The model under review builds one solid part; all positions refer to its coordinate system, in mm. A direction names the side the tool comes from. Coordinates: 2 decimals unless noted, no trailing zeros. Loops run counter-clockwise (first coordinate to the right, second up) from the corner with the lowest first, then second, coordinate; pieces in that order, holes last. Notation, with made-up numbers: M -29,49.5 L -10,49.5 A22 ccw -10,72.5 Z; hole C 70,-9 d8. An arc over 180 degrees is marked long. Use CSV: the item, a comma, the result in double quotes. Start each with the question number.
Autodesk Inventor part; units mm, degrees
ref_plane "YZ Plane" through (0, 0, 0) normal (1, 0, 0) x (0, 1, 0)
ref_plane "XZ Plane" through (0, 0, 0) normal (0, 1, 0) x (-1, 0, 0)
ref_plane "XY Plane" through (0, 0, 0) normal (0, 0, 1) x (1, 0, 0)
sketch "スケッチ1" plane through (0, 0, 0) normal (0, 0, 1) x (1, 0, 0)
  line L0 (-28, -52.5) -> (28, -52.5) construction
  line L1 (28, -52.5) -> (28, 52.5) construction
  line L2 (28, 52.5) -> (-28, 52.5) construction
  line L3 (-28, 52.5) -> (-28, -52.5) construction
  line L4 (-28, -52.5) -> (28, 52.5) construction
  line L5 (28, -52.5) -> (-28, 52.5) construction
  line L6 (-28, 39.6) -> (-28, 52.5)
  line L7 (-28, 52.5) -> (28, 52.5)
  line L8 (28, 52.5) -> (28, 39.6)
  line L9 (-28, 37.5) -> (-33, 37.5)
  line L10 (-33, 37.5) -> (-33, -37.5)
  line L11 (-33, -37.5) -> (-28, -37.5)
  line L12 (-28, -39.6) -> (-28, -52.5)
  line L13 (-28, -52.5) -> (28, -52.5)
  line L14 (28, -52.5) -> (28, -39.6)
  line L15 (28, 37.5) -> (33, 37.5)
  line L16 (33, 37.5) -> (33, -37.5)
  line L17 (33, -37.5) -> (28, -37.5)
  arc A0 (-28, 37.5) -> (-28, 39.6) centre (-28, 38.55) ccw
  arc A1 (-28, -39.6) -> (-28, -37.5) centre (-28, -38.55) ccw
  arc A2 (28, -37.5) -> (28, -39.6) centre (28, -38.55) ccw
  line L18 (0, 0) -> (0, 52.5) construction
  line L19 (0, 0) -> (28, 0) construction
  arc A3 (28, 39.6) -> (28, 37.5) centre (28, 38.55) ccw
  line L20 (-24.5, 44.5) -> (24.5, 44.5) construction
  line L21 (24.5, 44.5) -> (24.5, -13.5) construction
  line L22 (24.5, -13.5) -> (-24.5, -13.5) construction
  line L23 (-24.5, -13.5) -> (-24.5, 44.5) construction
  line L24 (-24.5, 44.5) -> (24.5, -13.5) construction
  line L25 (24.5, 44.5) -> (-24.5, -13.5) construction
  circle A4 centre (-24.5, 44.5) radius 1.04
  circle A5 centre (-24.5, -13.5) radius 1.04
  circle A6 centre (24.5, -13.5) radius 1.04
  circle A7 centre (24.5, 44.5) radius 1.04
  line L26 (-22, -27.5) -> (-17, -27.5) construction
  line L27 (-17, -27.5) -> (-17, -42.5) construction
  line L28 (-17, -42.5) -> (-22, -42.5) construction
  line L29 (-22, -42.5) -> (-22, -27.5) construction
  circle A8 centre (-19.5, -21.5) radius 1.55
  circle A9 centre (-19.5, -48.5) radius 1.55
  line L30 (-17, -35) -> (-22, -35) construction
  line L31 (-22, -17.5) -> (-17, -17.5) construction
  line L32 (-17, -17.5) -> (-17, -52.5) construction
  line L33 (-17, -52.5) -> (-22, -52.5) construction
  line L34 (-22, -52.5) -> (-22, -17.5) construction
  circle A10 centre (-19.5, -48.5) radius 3 construction
  line L35 (-16.95, -27.45) -> (-22.05, -27.45)
  line L36 (-22.05, -27.45) -> (-22.05, -42.55)
  line L37 (-22.05, -42.55) -> (-16.95, -42.55)
  line L38 (-16.95, -42.55) -> (-16.95, -27.45)
  circle A11 centre (-22.05, -28.5) radius 1.05
  circle A12 centre (-16.95, -28.5) radius 1.05
  circle A13 centre (-22.05, -41.5) radius 1.05
  circle A14 centre (-16.95, -41.5) radius 1.05
  circle A15 centre (19.5, -21.5) radius 1.55
  circle A16 centre (19.5, -48.5) radius 1.55
  line L39 (16.95, -27.45) -> (22.05, -27.45)
  line L40 (22.05, -27.45) -> (22.05, -42.55)
  line L41 (22.05, -42.55) -> (16.95, -42.55)
  line L42 (16.95, -42.55) -> (16.95, -27.45)
  circle A17 centre (22.05, -28.5) radius 1.05
  circle A18 centre (16.95, -28.5) radius 1.05
  circle A19 centre (22.05, -41.5) radius 1.05
  circle A20 centre (16.95, -41.5) radius 1.05
  point P0 (0, 15.5)
  point P1 (0, 15.5)
  point P2 (0, 0)
  point P3 (-19.5, -35)
  point P4 (-19.5, -17.5)
  dimension "d93" = 2.1
  dimension "d9" = 56
  dimension "d12" = 105
  dimension "d13" = 15
  dimension "d39" = 15
  dimension "d40" = 1.05
  dimension "d41" = 5
  dimension "d52" = 2.08
  dimension "d53" = 49
  dimension "d54" = 58
  dimension "d55" = 8
  dimension "d73" = 35
  dimension "d83" = 5
  dimension "d87" = 3.1
  dimension "d88" = 10
  dimension "d89" = 27
  dimension "d90" = 6
  dimension "d91" = 22
  dimension "d92" = 0.05
extrude "押し出し1" add sketch "スケッチ1" along normal blind 5
sketch "スケッチ2" plane through (0, 0, 5) normal (0, 0, 1) x (1, 0, 0)
  line L0 (-28, 52.5) -> (-28, 39.6)
  line L1 (28, 52.5) -> (-28, 52.5)
  line L2 (-67.7785, 43.014) -> (-28, 43.014)
  line L3 (-28, 43.014) -> (-28, -43.014)
  line L4 (-28, -43.014) -> (-67.7785, -43.014)
  line L5 (-67.7785, -43.014) -> (-67.7785, 43.014)
  line L6 (67.7785, 43.014) -> (28, 43.014)
  line L7 (28, 43.014) -> (28, -43.014)
  line L8 (28, -43.014) -> (67.7785, -43.014)
  line L9 (67.7785, -43.014) -> (67.7785, 43.014)
  line L10 (0, 0) -> (0, 52.5) construction
  line L11 (0, 0) -> (33, 0) construction
  line L12 (33, 37.5) -> (33, -37.5) construction
extrude "押し出し2" cut sketch "スケッチ2" against normal blind 2.5
sketch "スケッチ5" plane through (0, 0, 0) normal (0, 0, -1) x (-1, 0, 0)
  circle A0 centre (-24.5, 44.5) radius 1.04
  circle A1 centre (-24.5, 44.5) radius 1.04
  circle A2 centre (24.5, 44.5) radius 1.04
  circle A3 centre (24.5, 44.5) radius 1.04
  circle A4 centre (24.5, -13.5) radius 1.04
  circle A5 centre (24.5, -13.5) radius 1.04
  circle A6 centre (-24.5, -13.5) radius 1.04
  circle A7 centre (-24.5, -13.5) radius 1.04
  circle A8 centre (-19.5, -21.5) radius 1.55
  circle A9 centre (-19.5, -21.5) radius 1.55
  circle A10 centre (19.5, -21.5) radius 1.55
  circle A11 centre (19.5, -21.5) radius 1.55
  circle A12 centre (-19.5, -48.5) radius 1.55
  circle A13 centre (-19.5, -48.5) radius 1.55
  circle A14 centre (19.5, -48.5) radius 1.55
  circle A15 centre (19.5, -48.5) radius 1.55
  point P0 (0, 0)
extrude "押し出し5" add sketch "スケッチ5" against normal up to surface (5 mm away)
equation "\"d12\" = d19"
equation "\"d13\" = d26"
equation "\"d39\" = d27"
equation "\"d55\" = d69"
equation "\"d73\" = d1_1_2 + 2 * d2_1"
equation "\"d88\" = d2_1"
properties part number "コックピット_2_サブフレーム_1" material "アセタール樹脂、黒"
1. For faces 1 (the flat face through (0, 1, 5)), 2 (the flat face through (30, 1, 2.5)), 3 (the flat face through (-30, 37.5, 1)), 4 (the flat face through (-31, -37.5, 1)), 5 (the cylindrical face through (-23.1, -41.5, 2.5)), list the 3-axis set-ups (+Z, -Z, +X, -X, +Y, -Y) from which the entire face can be reached by the end or side of a thin tool; tool diameter is ignored.
2. Insertion check: pin 1 Ø1.5 at (x, y) = (30.5, -2.5) entering from +Z; pin 2 Ø2.5 at (y, z) = (43, 1.5) entering from +X; pin 3 Ø1.5 at (y, z) = (-46.5, 3.5) entering from -X. Each pin has a flat end and moves straight along its axis. Give the tip position at first contact, or say it passes through.
3. Draft analysis for pull direction Y (two halves, no side actions). For faces 6 (the flat face through (-33, 1, 1)), 7 (the cylindrical face through (-26.95, -38.53, 2.46)), 8 (the flat face through (30, 37.5, 1)), 9 (the flat face through (-20, -42.55, 2)), state which applies: released by +Y, released by -Y, zero draft, split by the parting line, or undercut.
4. Add section C-C (y = -25.5). Write out the cut boundary in (x, z).
5. Add section B-B (y = -41.5). Write out the cut boundary in (x, z).
6. To check wall thickness, follow line 1 along X through (y, z) = (-37, 0.4); line 2 along Y through (x, z) = (21.5, 2.85); line 3 along X through (y, z) = (-29, 0.8). State the ranges of each line that lie inside material, in increasing order.
7. Add section D-D (y = 38.55). Write out the cut boundary in (x, z).
8. Add section A-A (z = 0.95). Give the number of separate pieces and of enclosed holes in the cut face, plus the area to 3 significant figures.
Solved:
1,face 1,"+Z, +X, -X, +Y, -Y"
1,face 2,"+Z, +X, +Y, -Y"
1,face 3,"+Z, -Z, -X, +Y"
1,face 4,"+Z, -Z, -X, -Y"
1,face 5,"+Z, -Z"
2,pin 1,"stops at z = 2.5"
2,pin 2,"stops at x = 28"
2,pin 3,"stops at x = -28"
3,face 6,"zero draft"
3,face 7,"undercut"
3,face 8,"released by +Y"
3,face 9,"undercut"
4,outline,"M -33,0 L 33,0 L 33,2.5 L 28,2.5 L 28,5 L -28,5 L -28,2.5 L -33,2.5 Z"
5,outline,"M -28,0 L -23.1,0 L -23.1,5 L -28,5 Z; M -15.9,0 L 15.9,0 L 15.9,5 L -15.9,5 Z; M 23.1,0 L 28,0 L 28,5 L 23.1,5 Z"
6,line 1,"x = -33 to -22.05, -16.95 to 16.95, 22.05 to 33"
6,line 2,"y = -52.5 to -42.55, -27.45 to 52.5"
6,line 3,"x = -33 to -22.97, -16.03 to 16.03, 22.97 to 33"
7,outline,"M -26.95,0 L 26.95,0 L 26.95,5 L -26.95,5 Z"
8,separate pieces,"1"
8,enclosed holes,"2"
8,area,"6,460 mm^2"
